Check sheet for the modelled part. Datum: model origin and axes. Units: mm. A direction names the side the tool comes from. Give positions to 0.01 mm unless a question says otherwise; leave off trailing zeros. Write each loop counter-clockwise with the first axis right and the second up, starting at its lowest first coordinate (ties: lowest second). Pieces come first, ordered by that corner, then holes.
from build123d import *

# Parameters (mm, degrees)
SKETCH044_W     = 6
SKETCH044_H     = 6
PAD022_DEPTH    = 7
SKETCH046_R     = 1.25
POCKET013_DEPTH = 5.6
SKETCH047_R     = 1.25
PAD024_DEPTH    = 4.75


with BuildPart() as part:
    # Sketch044 → Pad022 (new body)
    with BuildSketch(Plane(origin=(-25.08, 0, 0), x_dir=(1, 0, 0), z_dir=(0, -1, 0))):
        with Locations((145, 14)):
            Rectangle(SKETCH044_W, SKETCH044_H)
    extrude(amount=-PAD022_DEPTH)

    # Sketch046 (on Face5 of Pad022) → Pocket013 (cut)
    with BuildSketch(Plane.XZ):
        with Locations((119.92, 14)):
            Circle(SKETCH046_R)
    extrude(amount=-POCKET013_DEPTH, mode=Mode.SUBTRACT)

    # Sketch047 → Pad024 (join)
    with BuildSketch(Plane(origin=(0, 0, 11), x_dir=(1, 0, 0), z_dir=(0, 0, -1))):
        with Locations((119.92, -3.5)):
            Circle(SKETCH047_R)
    extrude(amount=PAD024_DEPTH)


with BuildPart() as part_1:
    # Body009 placement: moved
    add(part.part.moved(Location((0, 11, 0))))


solid = part_1.part
1) Draft check along Z on faces 1 (the cylindrical face through (121.11, 13.76, 14.38)), 2 (the flat face through (116.92, 14, 14)), 3 (the flat face through (120, 14, 17)). Enter one of: +Z half, -Z half, draft (parallel to the pull), parting line (faces both ways), or undercut.
2) Gauge pin test, flat ends, axial feed: pin 1 (1.5 mm diameter, centred on x = 121.5, z = 8.5, fed in from +Y); pin 2 (2 mm diameter, centred on x = 119.5, z = 14, fed in from -Y). Record the tip position at first contact, or that the pin passes through.
3) Sectioned sample at A-A on y = 15.5. Record the boundary of the cut face in (x, z), then the cut area to 3 significant figures.
4) Sectioned sample at C-C on z = 14. Record the boundary of the cut face in (x, y), then the cut area to 3 significant figures.
5) Access from +Z, -Z, +X, -X, +Y, -Y to the whole of each face (thin tool, end or side, straight path). Record for faces 4 (the flat face through (122.92, 14, 14)), 5 (the flat face through (118.5, 14.5, 11)), 6 (the flat face through (120, 16.6, 14)).
6) Scan lines: L1, parallel to Z at x = 119.92, y = 13.1; L2, parallel to Z at x = 119.92, y = 15.25; L3, parallel to Z at x = 121.65, y = 15.25. Record each from-to range of solid material in increasing order.
7) Sectioned sample at B-B on x = 119.92. Record the boundary of the cut face in (y, z), then the cut area to 3 significant figures.
8) Sectioned sample at D-D on y = 14.5. Record the boundary of the cut face in (x, z), then the cut area to 3 significant figures.
Answers below:
1. face 1: undercut
1. face 2: draft
1. face 3: +Z half
2. pin 1: stops at y = 15.43
2. pin 2: stops at y = 11
3. outline: (116.92, 11) - (119.17, 11) - (119.17, 6.25) - (120.67, 6.25) - (120.67, 11) - (122.92, 11) - (122.92, 17) - (116.92, 17) - close; hole circle Ø2.5 at (119.92, 14)
3. area: 38.2 mm2
4. outline: (116.92, 11) - (118.67, 11) - (118.67, 16.6) - (121.17, 16.6) - (121.17, 11) - (122.92, 11) - (122.92, 18) - (116.92, 18) - close
4. area: 28.0 mm2
5. face 4: +Z, -Z, +X, +Y, -Y
5. face 5: -Z
5. face 6: -Y
6. L1: z = 11 to 12.75, 15.25 to 17
6. L2: z = 6.25 to 12.75, 15.25 to 17
6. L3: z = 11 to 17
7. outline: (11, 11) - (13.25, 11) - (13.25, 6.25) - (15.75, 6.25) - (15.75, 11) - (18, 11) - (18, 17) - (11, 17) - (11, 15.25) - (16.6, 15.25) - (16.6, 12.75) - (11, 12.75) - close
7. area: 39.9 mm2
8. outline: (116.92, 11) - (118.67, 11) - (118.67, 6.25) - (121.17, 6.25) - (121.17, 11) - (122.92, 11) - (122.92, 17) - (116.92, 17) - close; hole circle Ø2.5 at (119.92, 14)
8. area: 43.0 mm2
